For this review, take the finished solid that the model builds, in its own axes (mm). A direction names the side the tool comes from. Round coordinates to 2 decimals unless told otherwise and drop trailing zeros. Order: outer loops, then holes, each group sorted by start corner. A loop starts at its lowest first (then second) coordinate and runs counter-clockwise, first axis right, second up. Notation, with made-up numbers: (-8.75, 62) - (42.25, 62) arc R19 cw to (42.25, 96) - close; hole circle Ø1 at (-16.5, -8). An arc over 180 degrees is marked (long way). One line per item, written item: value.
```python
from build123d import *

# Parameters (mm, degrees)
SKETCH3_W           = 38.1
SKETCH3_H           = 38.1
BOSS_EXTRUDE2_DEPTH = 38.1
SKETCH5_R           = 10
CUT_EXTRUDE1_DEPTH  = 967.362983045
SKETCH7_W           = 7.62
SKETCH7_H           = 116.34084036
CUT_EXTRUDE2_DEPTH  = 60


with BuildPart() as part:
    # Sweep1: sweep along a path in Sketch2
    with BuildLine(Plane(origin=(0, 0, 0), x_dir=(0, 0, -1), z_dir=(1, 0, 0))) as sweep1_path:
        ThreePointArc((862.5, 0), (856.407116711, 23.91997287), (839.613395916, 42.010281621))
        Line((839.613395916, 42.010281621), (385.566979579, 335.051408107))
        ThreePointArc((385.566979579, 335.051408107), (130.40013565, 344.535583556), (0, 125))
    # Sketch3 → Sweep1 (sweep)
    with BuildSketch(Plane(origin=(0, 0, 0), x_dir=(1, 0, 0), z_dir=(0, 1, 0))):
        with Locations((0, 862.5)):
            Rectangle(SKETCH3_W, SKETCH3_H)
    sweep(path=sweep1_path.line)

    # Sketch4 → Boss-Extrude2 (add)
    with BuildSketch(Plane(origin=(19.05, 0, 0), x_dir=(0, 0, -1), z_dir=(1, 0, 0))):
        with BuildLine():
            ThreePointArc((22.92164625, 144.354537793), (20.985722139, 147.926611635), (20.630635597, 151.974009223))
            ThreePointArc((20.630635597, 151.974009223), (19.44549754, 138.510140473), (19.05, 125))
            Line((19.05, 125), (10, 125))
            ThreePointArc((10, 125), (0, 115), (-10, 125))
            Line((-10, 125), (-19.05, 125))
            ThreePointArc((-19.05, 125), (-18.685251714, 139.004928115), (-17.591995826, 152.971883559))
            ThreePointArc((-17.591995826, 152.971883559), (-18.567549982, 149.591749406), (-20.65335375, 146.758652966))
            ThreePointArc((-20.65335375, 146.758652966), (-1.652643385, 95.04555509), (22.92164625, 144.354537793))
        make_face()
    extrude(amount=-BOSS_EXTRUDE2_DEPTH)

    # Sketch5 → Cut-Extrude1 (cut, through all)
    with BuildSketch(Plane(origin=(19.05, 0, 0), x_dir=(0, 0, -1), z_dir=(1, 0, 0))):
        with Locations((0, 125)):
            Circle(SKETCH5_R)
    extrude(amount=-CUT_EXTRUDE1_DEPTH, mode=Mode.SUBTRACT)

    # Sketch7 → Cut-Extrude2 (cut)
    with BuildSketch(Plane(origin=(0, 95, 0), x_dir=(-1, 0, 0), z_dir=(0, -1, 0))):
        with Locations((-15.24, -0.743263463)):
            Rectangle(SKETCH7_W, SKETCH7_H)
        with Locations((0, -0.743263463)):
            Rectangle(SKETCH7_W, SKETCH7_H)
        with Locations((15.24, -0.743263463)):
            Rectangle(SKETCH7_W, SKETCH7_H)
    extrude(amount=-CUT_EXTRUDE2_DEPTH, mode=Mode.SUBTRACT)


solid = part.part
```
Item 1: Machinability: for faces 4 (the flat face through (11.43, 138, 0)), 5 (the flat face through (-11.43, 138, 0)), 6 (the flat face through (-0.267, 174.576, -599.082)), 7 (the flat face through (-3.81, 138, 0)), 8 (the cylindrical face through (-7.567, 95.115, 2.628)), which of the approach directions +Z, -Z, +X, -X, +Y, -Y give a long, thin tool a straight path to every point of the face, cutting with its end or side? Answer none if there is none.
Returned:
face 4: +Z, +X, -Y
face 5: +Z, -X, -Y
face 6: +X, -X, -Y
face 7: +Z, -Y
face 8: +X, -X
Item 2: Take a section at B-B (y = 250.5). Write out the cut boundary in (x, z), plus the area to 3 significant figures.
Returned:
outline: (-19.05, -551.7) - (19.05, -551.7) - (19.05, -481.44) - (-19.05, -481.44) - close; (-19.05, -56.12) - (19.05, -56.12) - (19.05, -12.01) - (-19.05, -12.01) - close
area: 4,360 mm^2
Item 3: For P1, Ø18, axis at y = 118.5, z = -6.5, coming from the -X side; P2, Ø3, axis at x = -3, z = -610.5, coming from the +Y side; P3, Ø4, axis at x = 14.5, z = 2, coming from the -Y side; P4, Ø2, axis at y = 250, z = -555.5, coming from the -X side, all flat-tipped, find the tip position at first contact; note any pin that passes through.
Returned:
P1: x = -11.43
P2: y = 213.52
P3: y = 155
P4: through
Item 4: The part is to be moulded in two halves that separate along X. For faces 1 (the flat face through (19.05, 286, -430)), 2 (the cylindrical face through (0.27, 335.3, -154.54)), 3 (the flat face through (3.81, 138, 0)), say which applies: +X half, -X half, draft (parallel to the pull), parting line (faces both ways), or undercut.
Returned:
face 1: +X half
face 2: draft
face 3: undercut
Item 5: Take a section at C-C (y = 125). Write out the cut boundary in (x, z).
Returned:
outline: (-19.05, -746.16) - (19.05, -746.16) - (19.05, -675.9) - (-19.05, -675.9) - close; (-11.43, -30) - (-3.81, -30) - (-3.81, -10) - (-11.43, -10) - close; (-11.43, 10) - (-3.81, 10) - (-3.81, 30) - (-11.43, 30) - close; (3.81, -30) - (11.43, -30) - (11.43, -10) - (3.81, -10) - close; (3.81, 10) - (11.43, 10) - (11.43, 30) - (3.81, 30) - close
Item 6: Take a section at A-A (z = 0). Write out the cut boundary in (x, y).
Returned:
outline: (-19.05, 155) - (-11.43, 155) - (-11.43, 135) - (-3.81, 135) - (-3.81, 155) - (3.81, 155) - (3.81, 135) - (11.43, 135) - (11.43, 155) - (19.05, 155) - (19.05, 224.44) - (-19.05, 224.44) - close; (-11.43, 95) - (-3.81, 95) - (-3.81, 115) - (-11.43, 115) - close; (3.81, 95) - (11.43, 95) - (11.43, 115) - (3.81, 115) - close
Item 7: Take a section at D-D (y = 331.5). Write out the cut boundary in (x, z).
Returned:
outline: (-19.05, -426.2) - (19.05, -426.2) - (19.05, -353.42) - (-19.05, -353.42) - close; (-19.05, -146.58) - (19.05, -146.58) - (19.05, -77.53) - (-19.05, -77.53) - close
Item 8: Wall thickness on line 1 (Z direction, x = 11, y = 121); line 2 (Z direction, x = -4.5, y = 131.5); line 3 (Z direction, x = 9.5, y = 285): over which ranges is each line inside the solid? List them lowest first.
Returned:
line 1: -752.35 to -682.09, -29.73 to -9.17, 9.17 to 29.73
line 2: -736.09 to -665.83, -29.29 to -7.6, 7.6 to 29.29
line 3: -498.25 to -427.99, -83.45 to -33.69
